Source: three-view drawing plus pictorial views. Frame: mm from the lowest corner of the part. Give positions to 0.01 mm unless a question says otherwise; leave off trailing zeros. Loops run counter-clockwise (first coordinate to the right, second up) from the corner with the lowest first, then second, coordinate; pieces in that order, holes last.
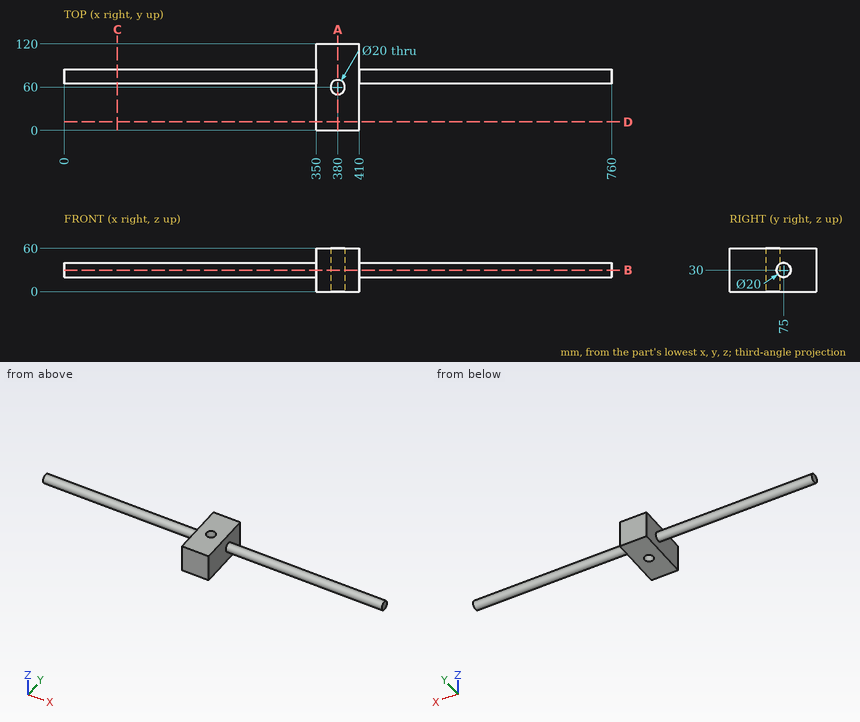
(1) Ray query, probe 1 along X at (y, z) = (60, 19.5); probe 2 along Y at (x, z) = (380, 21.5); probe 3 along X at (y, z) = (30, 19.5). Return the intervals inside material, ascending.
Values follow:
probe 1: x = 350 to 370, 390 to 410
probe 2: y = 0 to 50, 70 to 120
probe 3: x = 350 to 410
(2) Cut plane C-C (x = 74). Return the cut outline in (y, z), and give its area (3 significant figures).
Values follow:
outline: circle Ø20 at (75, 30)
area: 314 mm2
(3) Cut plane A-A (x = 380). Return the cut outline in (y, z), and give its area (3 significant figures).
Values follow:
outline: (0, 0) - (50, 0) - (50, 60) - (0, 60) - close; (70, 0) - (120, 0) - (120, 60) - (70, 60) - close
area: 6,000 mm2
(4) Cut plane D-D (y = 12). Return the cut outline in (x, z).
Values follow:
outline: (350, 0) - (410, 0) - (410, 60) - (350, 60) - close
(5) Cut plane B-B (z = 30). Return the cut outline in (x, y), and give its area (3 significant figures).
Values follow:
outline: (0, 65) - (350, 65) - (350, 0) - (410, 0) - (410, 65) - (760, 65) - (760, 85) - (410, 85) - (410, 120) - (350, 120) - (350, 85) - (0, 85) - close; hole circle Ø20 at (380, 60)
area: 20,900 mm2
(6) Pin query (flat end, axial travel): pin 1 Ø10 at (y, z) = (100, 20.5) entering from +X; pin 2 Ø12 at (x, y) = (115.5, 85.5) entering from -Z; pin 3 Ø2 at (x, y) = (295, 76.5) entering from -Z. Return the tip coordinate at first contact, or that it passes through.
Values follow:
pin 1: stops at x = 410
pin 2: stops at z = 21.07
pin 3: stops at z = 20.01
